Could you check a few things on this model? Use its own coordinates, in mm. A direction names the side the tool comes from. Coordinates: 2 decimals unless noted, no trailing zeros. Loops run counter-clockwise (first coordinate to the right, second up) from the corner with the lowest first, then second, coordinate; pieces in that order, holes last. Notation, with made-up numbers: (62, 8) - (76, 8) arc R19 ccw to (76, 19) - close; hole circle Ø3 at (10, 30). An arc over 180 degrees is marked (long way). One line per item, written item: value. Start each with the question number.
(1) On a 3-axis mill with a long thin cutter (end or side, diameter ignored), from which of +Z, -Z, +X, -X, +Y, -Y can I reach the whole of each face in a straight line? I mean faces 1 (the face through (7.62, -3.16, 24.93)), 2 (the face through (-0.228, -10.494, 27.735)). Say none if no direction works.
(2) If I drill on line 1 along Y through (x, z) = (-4, 28); line 2 along Y through (x, z) = (-6.75, 5.5); line 3 along X through (y, z) = (1, 11), over which ranges is the centre line in solid material (lowest first)? Write a range as from..to.
(3) If we mould it in two halves opening along Z, with no side actions, what happens to faces 3 (the face through (4, 7.4, 30)), 4 (the face through (3.815, -11.91, 27.201)), 5 (the face through (2, -13, 25))? For each: pulls with the +Z half, pulls with the -Z half, needs draft (parallel to the pull), parting line crosses it, or undercut.
(4) If we section it at A-A on y = 0: Write out the boundary of the cut face in (x, z).
(5) If we section it at C-C on z = 4.5: Write out the boundary of the cut face in (x, y) (3 decimals).
(6) I'm going to push flat-ended pins straight in: P1, Ø1.5, axis at x = 0.5, z = 16.5, coming from the +Y side; P2, Ø12, axis at y = -4.5, z = 12, coming from the -X side; P3, Ø5, axis at y = -5.5, z = 18.5, coming from the -X side; P4, Ø12, axis at x = 6.5, z = 24, coming from the -Y side. Where does each tip first touch, or does it pass through?
(7) If we section it at D-D on z = 15.5: Write out the boundary of the cut face in (x, y) (3 decimals).
(8) If we section it at B-B on z = 26: Write out the boundary of the cut face in (x, y).
```python
from build123d import *

# Parameters (mm, degrees)
CYLINDER035_R     = 11
CYLINDER035_DEPTH = 10
CYLINDER036_R     = 8.25
CYLINDER036_DEPTH = 10
CYLINDER058_R     = 4
CYLINDER058_DEPTH = 4
CYLINDER059_R     = 1.75
CYLINDER059_DEPTH = 6


with BuildPart() as part:
    # Cone001 → Cone001 (revolve)
    with BuildSketch(Plane.XZ):
        Polygon((0, 0), (13, 0), (11, 20), (0, 20), align=None)
    revolve(axis=Axis((0, 0, 0), (0, 0, 1)))

    # Cone002 → Cone002 (revolve, cut)
    with BuildSketch(Plane.XZ):
        Polygon((0, 0), (11.25, 0), (8.25, 20), (0, 20), align=None)
    revolve(axis=Axis((0, 0, 0), (0, 0, 1)), mode=Mode.SUBTRACT)

    # Cylinder035 → Cylinder035 (join)
    with BuildSketch(Plane.XY.offset(20)):
        Circle(CYLINDER035_R)
    extrude(amount=CYLINDER035_DEPTH)

    # Cylinder036 → Cylinder036 (cut)
    with BuildSketch(Plane.XY.offset(20)):
        Circle(CYLINDER036_R)
    extrude(amount=CYLINDER036_DEPTH, mode=Mode.SUBTRACT)

    # Cylinder058 → Cylinder058 (join)
    with BuildSketch(Plane(origin=(0, -9, 26), x_dir=(1, 0, 0), z_dir=(0, -1, 0))):
        Circle(CYLINDER058_R)
    extrude(amount=CYLINDER058_DEPTH)

    # Cylinder059 → Cylinder059 (cut)
    with BuildSketch(Plane(origin=(0, -7, 26), x_dir=(1, 0, 0), z_dir=(0, -1, 0))):
        Circle(CYLINDER059_R)
    extrude(amount=CYLINDER059_DEPTH, mode=Mode.SUBTRACT)


solid = part.part
```
Values:
1. face 1: +Z, -Z
1. face 2: -Y
2. line 1: y = -10.25..-7.22, 7.22..10.25
2. line 2: y = -10.46..-7.94, 7.94..10.46
2. line 3: x = -11.86..-9.55, 9.55..11.86
3. face 3: pulls with the +Z half
3. face 4: undercut
3. face 5: needs draft
4. outline: (-13, 0) - (-11.25, 0) - (-8.25, 20) - (-8.25, 30) - (-11, 30) - (-11, 20) - close; (8.25, 20) - (11.25, 0) - (13, 0) - (11, 20) - (11, 30) - (8.25, 30) - close
5. outline: circle Ø25.1 at (0, 0); hole circle Ø21.15 at (0, 0)
6. P1: stops at y = 11.42
6. P2: stops at x = -12.25
6. P3: stops at x = -10.78
6. P4: stops at y = -13
7. outline: circle Ø22.9 at (0, 0); hole circle Ø17.85 at (0, 0)
8. outline: (-4, -13) - (-1.75, -13) - (-1.75, -8.06) arc R8.25 cw (long way) to (1.75, -8.06) - (1.75, -13) - (4, -13) - (4, -10.25) arc R11 ccw (long way) to (-4, -10.25) - close
